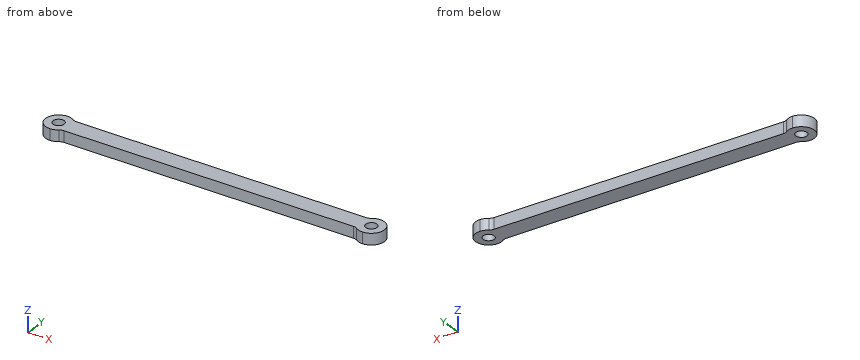
from build123d import *
from build123d.topology import SkipClean

# Parameters (mm, degrees)
SKETCH_1_R          = 1.5
EXTRUDE_1_DEPTH     = 3
CUT_EXTRUDE_1_DEPTH = 89.619975175


with BuildPart() as part:
    # 草图1 → 凸台-拉伸1 (new body)
    with BuildSketch(Plane.XY):
        with BuildLine():
            Line((0, 3.5), (85, 3.5))
            ThreePointArc((85, 3.5), (88.5, 0), (85, -3.5))
            Line((85, -3.5), (0, -3.5))
            ThreePointArc((0, -3.5), (-3.5, 0), (0, 3.5))
        make_face()
        Circle(SKETCH_1_R, mode=Mode.SUBTRACT)
        with Locations((85, 0)):
            Circle(SKETCH_1_R, mode=Mode.SUBTRACT)
    extrude(amount=EXTRUDE_1_DEPTH)

    # 草图2 → 切除-拉伸1 (cut, through all)
    with SkipClean():  # the faces are left unmerged after this step: merging them gives an invalid solid
        with BuildSketch(Plane.XY.offset(3)):
            with BuildLine():
                Line((3.16227766, 2.5), (81.83772234, 2.5))
                ThreePointArc((81.83772234, 2.5), (82.440745029, 2.593074822), (82.987641489, 2.863636364))
                ThreePointArc((82.987641489, 2.863636364), (83.944710294, 3.337119062), (85, 3.5))
                Line((85, 3.5), (0, 3.5))
                ThreePointArc((0, 3.5), (1.055289706, 3.337119062), (2.012358511, 2.863636364))
                ThreePointArc((2.012358511, 2.863636364), (2.559254971, 2.593074822), (3.16227766, 2.5))
            make_face()
            with BuildLine():
                Line((3.16227766, -2.5), (81.83772234, -2.5))
                ThreePointArc((81.83772234, -2.5), (82.440745029, -2.593074822), (82.987641489, -2.863636364))
                ThreePointArc((82.987641489, -2.863636364), (83.944710294, -3.337119062), (85, -3.5))
                Line((85, -3.5), (0, -3.5))
                ThreePointArc((0, -3.5), (1.055289706, -3.337119062), (2.012358511, -2.863636364))
                ThreePointArc((2.012358511, -2.863636364), (2.559254971, -2.593074822), (3.16227766, -2.5))
            make_face()
        extrude(amount=-CUT_EXTRUDE_1_DEPTH, mode=Mode.SUBTRACT)


solid = part.part
Input: part model. Units: mm. Frame: model coordinates. Coordinates: 2 decimals unless noted, no trailing zeros. Order: outer loops, then holes, each group sorted by start corner. A loop starts at its lowest first (then second) coordinate and runs counter-clockwise, first axis right, second up.
1. Ray query, line 1 along X through (y, z) = (-1, 2.3); line 2 along Y through (x, z) = (85, 1.3); line 3 along X through (y, z) = (0.75, 0.5). Return the intervals inside material, ascending.
Checked values:
line 1: x = -3.35 to -1.12, 1.12 to 83.88, 86.12 to 88.35
line 2: y = -3.5 to -1.5, 1.5 to 3.5
line 3: x = -3.42 to -1.3, 1.3 to 83.7, 86.3 to 88.42
2. Contact query for a flat-ended pin moving along its axis: P1, Ø1.5, axis at x = 53, z = 1.5, coming from the -Y side. Output: stop coordinate, or through.
Checked values:
P1: stops at y = -2.5
3. Cut plane B-B, the plane z = 2.35. Return loops of the section in (x, y).
Checked values:
outline: (2.01, -2.86) arc R2 cw to (3.16, -2.5) - (81.84, -2.5) arc R2 cw to (82.99, -2.86) arc R3.5 ccw (long way) to (82.99, 2.86) arc R2 cw to (81.84, 2.5) - (3.16, 2.5) arc R2 cw to (2.01, 2.86) arc R3.5 ccw (long way) to start; hole circle Ø3 at (0, 0); hole circle Ø3 at (85, 0)
4. Cut plane A-A, the plane y = 0. Return loops of the section in (x, z).
Checked values:
outline: (-3.5, 0) - (-1.5, 0) - (-1.5, 3) - (-3.5, 3) - close; (1.5, 0) - (83.5, 0) - (83.5, 3) - (1.5, 3) - close; (86.5, 0) - (88.5, 0) - (88.5, 3) - (86.5, 3) - close
5. Cut plane C-C, the plane x = 15.5. Return loops of the section in (y, z), plus the area to 3 significant figures.
Checked values:
outline: (-2.5, 0) - (2.5, 0) - (2.5, 3) - (-2.5, 3) - close
area: 15.0 mm2
